```python
from build123d import *

# Parameters (mm, degrees)
SALIENTE_EXTRUIR1_DEPTH         = 10
REDONDEO2_R                     = 5
REDONDEO3_R                     = 5
REDONDEO5_R                     = 2
TALADRO_ROSCADO_M51_D           = 5.5
TALADRO_ROSCADO_M51_CBORE_D     = 10
TALADRO_ROSCADO_M51_CBORE_DEPTH = 5.4


with BuildPart() as part:
    # Croquis1 → Saliente-Extruir1 (new body)
    with BuildSketch(Plane(origin=(0, 0, 0), x_dir=(1, 0, 0), z_dir=(0, 1, 0))):
        Polygon((27.79756746, -8), (27.79756746, 47), (15.79756746, 47), (15.79756746, 72), (67.79756746, 72), (67.79756746, -8), align=None)
    extrude(amount=SALIENTE_EXTRUIR1_DEPTH)

    # Redondeo2
    redondeo2_edges = [part.edges().sort_by_distance(p)[0] for p in [
        (15.79756746, 5, -72),
        (67.79756746, 5, -72),
        (67.79756746, 5, 8),
        (27.79756746, 5, 8),
        (27.79756746, 5, -47),
        (15.79756746, 5, -47),
    ]]
    fillet(redondeo2_edges, radius=REDONDEO2_R)

    # Redondeo3
    redondeo3_edges = [part.edges().sort_by_distance(p)[0] for p in [
        (47.79756746, 10, 8),
        (27.79756746, 10, -19.5),
        (15.79756746, 10, -59.5),
        (21.79756746, 10, -47),
        (67.79756746, 10, -32),
        (41.79756746, 10, -72),
        (17.262033554, 10, -48.464466094),
        (66.333101366, 10, 6.535533906),
        (66.333101366, 10, -70.535533906),
        (17.262033554, 10, -70.535533906),
        (29.262033554, 10, 6.535533906),
        (26.333101366, 10, -45.535533906),
    ]]
    fillet(redondeo3_edges, radius=REDONDEO3_R)

    # Redondeo5
    redondeo5_edges = [part.edges().sort_by_distance(p)[0] for p in [
        (47.79756746, 0, 8),
        (15.79756746, 0, -59.5),
        (41.79756746, 0, -72),
        (67.79756746, 0, -32),
        (27.79756746, 0, -19.5),
        (21.79756746, 0, -47),
        (17.262033554, 0, -48.464466094),
        (66.333101366, 0, 6.535533906),
        (66.333101366, 0, -70.535533906),
        (17.262033554, 0, -70.535533906),
        (29.262033554, 0, 6.535533906),
        (26.333101366, 0, -45.535533906),
    ]]
    fillet(redondeo5_edges, radius=REDONDEO5_R)

    # Taladro roscado M51 (through all)
    with Locations(Plane(origin=(-0.50897812, 10, 14.967559644), x_dir=(-1, 0, 0), z_dir=(0, 1, 0))):
        with Locations((-56.30654558, -72.967559644), (-40.30654558, -72.967559644)):
            CounterBoreHole(TALADRO_ROSCADO_M51_D / 2, TALADRO_ROSCADO_M51_CBORE_D / 2, TALADRO_ROSCADO_M51_CBORE_DEPTH)


solid = part.part
```
The listing builds one solid part. Answer for the finished solid, in the listing's coordinates (mm). A direction names the side the tool comes from. Give positions to 0.01 mm unless a question says otherwise; leave off trailing zeros. Order: outer loops, then holes, each group sorted by start corner. A loop starts at its lowest first (then second) coordinate and runs counter-clockwise, first axis right, second up. Notation, with made-up numbers: M 69.5,-3 L 91.5,-3 A9 ccw 91.5,10 Z; hole C -6.5,34 d5. An arc over 180 degrees is marked long. Put each result on its own line as item: value. Start each with the question number.
Item 1: The part is cut by section B-B, the plane y = 3.75. Determine the outline of the cut face in (x, z), and give its area (3 significant figures).
Item 2: Flat-ended cylindrical pins translate along their axes: P1, Ø4, axis at y = 7.5, z = -57, coming from the +X side; P2, Ø6, axis at y = 2.5, z = -25, coming from the -X side; P3, Ø9, axis at x = 39.8, z = -58, coming from the +Y side. Find the tip coordinate at first contact, or state that the pin passes through.
Item 3: The part is cut by section A-A, the plane z = -58. Determine the outline of the cut face in (x, y), and give its area (3 significant figures).
Item 4: The part is cut by section D-D, the plane z = -14. Determine the outline of the cut face in (x, y), and give its area (3 significant figures).
Item 5: Which of the six approach directions +Z, -Z, +X, -X, +Y, -Y give full straight-line access (tool end or side, diameter ignored) to faces 4 (the face through (22, 9, -49)), 5 (the face through (22, 3, -47)), 6 (the face through (66.37, 3.52, 6.5)), 7 (the face through (37.6, 4.6, -60.2))?
Item 6: Find the intervals of material crossed by line 1 along X through (y, z) = (5, -38.5); line 2 along X through (y, z) = (8.5, -62.5); line 3 along X through (y, z) = (9, 1.5), in increasing order.
Item 7: For a pull along Z with two mould halves and no side action, classify faces 1 (the face through (17.301, 3.521, -48.426)), 2 (the face through (56.448, 7.338, -53.043)), 3 (the face through (28.4, 0.57, -19.82)) as +Z half, -Z half, draft (parallel to the pull), parting line (faces both ways), or undercut.
Item 8: The part is cut by section C-C, the plane x = 47. Determine the outline of the cut face in (y, z), and give its area (3 significant figures).
Answer key:
1. outline: M 15.8,-67 A5 ccw 20.8,-72 L 62.8,-72 A5 ccw 67.8,-67 L 67.8,3 A5 ccw 62.8,8 L 32.8,8 A5 ccw 27.8,3 L 27.8,-42 A5 cw 22.8,-47 L 20.8,-47 A5 ccw 15.8,-52 Z; hole C 39.8,-58 d5.5; hole C 55.8,-58 d5.5
1. area: 3,430 mm²
2. P1: stops at x = 67.77
2. P2: stops at x = 27.8
2. P3: stops at y = 4.6
3. outline: M 15.8,2 A2 ccw 17.8,0 L 37.05,0 L 37.05,4.6 L 34.8,4.6 L 34.8,10 L 20.8,10 A5 ccw 15.8,5 Z; M 42.55,0 L 53.05,0 L 53.05,4.6 L 50.8,4.6 L 50.8,10 L 44.8,10 L 44.8,4.6 L 42.55,4.6 Z; M 58.55,0 L 65.8,0 A2 ccw 67.8,2 L 67.8,5 A5 ccw 62.8,10 L 60.8,10 L 60.8,4.6 L 58.55,4.6 Z
3. area: 349 mm²
4. outline: M 27.8,2 A2 ccw 29.8,0 L 65.8,0 A2 ccw 67.8,2 L 67.8,5 A5 ccw 62.8,10 L 32.8,10 A5 ccw 27.8,5 Z
4. area: 388 mm²
5. face 4: +Z, -X, +Y
5. face 5: +Z, -X, +Y, -Y
5. face 6: +Z, +X, +Y, -Y
5. face 7: +Y
6. line 1: x = 27.8 to 67.8
6. line 2: x = 17.23 to 37.62, 41.98 to 53.62, 57.98 to 66.37
6. line 3: x = 29.8 to 65.8
7. face 1: +Z half
7. face 2: undercut
7. face 3: draft
8. outline: M 0,-70 A2 ccw 2,-72 L 5,-72 A5 ccw 10,-67 L 10,3 A5 ccw 5,8 L 2,8 A2 ccw 0,6 Z
8. area: 788 mm²
